Check sheet for the modelled part. Datum: model origin and axes. Units: mm. Round coordinates to 2 decimals unless told otherwise and drop trailing zeros. Write each loop counter-clockwise with the first axis right and the second up, starting at its lowest first coordinate (ties: lowest second). Pieces come first, ordered by that corner, then holes.
Item 1: Section check C-C, the plane z = -1. State how many separate pieces and enclosed holes the cut face has, plus the area to 3 significant figures.
Item 2: Release check for a two-part mould opening along X. For faces 1 (the flat face through (7, 4, 0)), 2 (the flat face through (-16, 2, 0)), 3 (the cylindrical face through (22.265, 2.028, 0.806)), 4 (the cylindrical face through (29.487, 2.028, -0.195)) record: pulls with the +X half, pulls with the -X half, needs draft (parallel to the pull), parting line crosses it, or undercut.
Item 3: Section check B-B, the plane y = 1.65. Record the cut outline in (x, z), plus the area to 3 significant figures.
Item 4: Material ranges on line 1 along X through (y, z) = (2.1, 0); line 2 along X through (y, z) = (2.8, 0); line 3 along X through (y, z) = (2.85, 3), recorded low to high.
Item 5: Depth check by flat-ended pin: pin 1 (2.5 mm diameter, centred on x = 21, z = 0, fed in from +Y). Enter the tip coordinate at first touch or a pass-through.
Item 6: Section check A-A, the plane x = 28. Record the cut outline in (y, z).
from build123d import *

# Parameters (mm, degrees)
SKETCH1_W           = 32
SKETCH1_H           = 12
BOSS_EXTRUDE1_DEPTH = 4
FILLET1_R           = 4
FILLET2_R           = 0.5
SKETCH3_W           = 12
SKETCH3_H           = 4
BOSS_EXTRUDE2_DEPTH = 15
SKETCH5_R           = 1.5
CUT_EXTRUDE1_DEPTH  = 32.827661054
FILLET4_R           = 1


with BuildPart() as part:
    # Sketch1 → Boss-Extrude1 (new body)
    with BuildSketch(Plane(origin=(0, 0, 0), x_dir=(1, 0, 0), z_dir=(0, 1, 0))):
        Rectangle(SKETCH1_W, SKETCH1_H)
    extrude(amount=BOSS_EXTRUDE1_DEPTH)

    # Sketch2 → Cut-Revolve1 (revolve, cut)
    with BuildSketch(Plane.XY):
        with BuildLine():
            Line((-10, 4), (-10, 0))
            Line((-10, 0), (-13.5, 0))
            ThreePointArc((-13.5, 0), (-14.031128874, 2), (-13.5, 4))
            Line((-13.5, 4), (-10, 4))
        make_face()
    revolve(axis=Axis((-10, 4, 0), (0, -1, 0)), mode=Mode.SUBTRACT)

    # Fillet1
    fillet1_edges = [part.edges().sort_by_distance(p)[0] for p in [
        (-16, 2, -6),
        (-16, 2, 6),
    ]]
    fillet(fillet1_edges, radius=FILLET1_R)

    # Fillet2
    fillet2_edges = [part.edges().sort_by_distance(p)[0] for p in [
        (-6.5, 4, 0),
        (-6.5, 0, 0),
    ]]
    fillet(fillet2_edges, radius=FILLET2_R)

    # Sketch3 → Boss-Extrude2 (add)
    with BuildSketch(Plane(origin=(16, 0, 0), x_dir=(0, 0, -1), z_dir=(1, 0, 0))):
        with Locations((0, 2)):
            Rectangle(SKETCH3_W, SKETCH3_H)
    extrude(amount=BOSS_EXTRUDE2_DEPTH)

    # Sketch5 → Cut-Extrude1 (cut, through all)
    with BuildSketch(Plane(origin=(0, 4, 0), x_dir=(1, 0, 0), z_dir=(0, 1, 0))):
        with Locations(Location((21, 0, 0), (0, 0, 270))):
            Circle(SKETCH5_R)
        with Locations(Location((28, 0, 0), (0, 0, 270))):
            Circle(SKETCH5_R)
    extrude(amount=-CUT_EXTRUDE1_DEPTH, mode=Mode.SUBTRACT)

    # Fillet4
    fillet4_edges = [part.edges().sort_by_distance(p)[0] for p in [
        (31, 2, 6),
        (31, 2, -6),
    ]]
    fillet(fillet4_edges, radius=FILLET4_R)


solid = part.part
Values found:
1. separate pieces: 4
1. enclosed holes: 0
1. area: 140 mm2
2. face 1: needs draft
2. face 2: pulls with the -X half
2. face 3: undercut
2. face 4: undercut
3. outline: (-16, -2) arc R4 ccw to (-12, -6) - (30, -6) arc R1 ccw to (31, -5) - (31, 5) arc R1 ccw to (30, 6) - (-12, 6) arc R4 ccw to (-16, 2) - close; hole circle Ø8.03 at (-10, 0); hole circle Ø3 at (21, 0); hole circle Ø3 at (28, 0)
3. area: 492 mm2
4. line 1: x = -16 to -14.03, -5.97 to 19.5, 22.5 to 26.5, 29.5 to 31
4. line 2: x = -16 to -13.95, -6.05 to 19.5, 22.5 to 26.5, 29.5 to 31
4. line 3: x = -15.87 to -12.55, -7.45 to 31
5. pin 1: passes through
6. outline: (0, -6) - (4, -6) - (4, -1.5) - (0, -1.5) - close; (0, 1.5) - (4, 1.5) - (4, 6) - (0, 6) - close
